Here's how the part is built. I have some questions about the finished solid (model axes, mm). Round coordinates to 2 decimals unless told otherwise and drop trailing zeros. Order: outer loops, then holes, each group sorted by start corner. A loop starts at its lowest first (then second) coordinate and runs counter-clockwise, first axis right, second up. Notation, with made-up numbers: (80.5, -17.5) - (93.5, -17.5) arc R21 ccw to (93.5, -9.5) - close; hole circle Ø6 at (82, 6.5). An arc over 180 degrees is marked (long way). Answer as a JSON object with one key per item and string values.
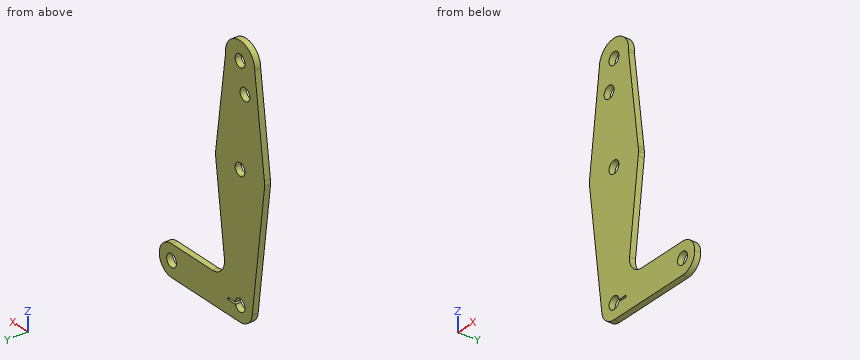
```python
from build123d import *

# Parameters (mm, degrees)
F0_R     = 3.175
F1_DEPTH = 3.048


with BuildPart() as f1:
    # F0 (on Front) → F1 (new body)
    with BuildSketch(Plane.XZ):
        with BuildLine():
            ThreePointArc((-9.525, 50.8), (-6.7351920908, 44.0648079092), (0, 41.275))
            ThreePointArc((0, 41.275), (6.3093081085, 43.6642970779), (9.4533014816, 49.6335026369))
            ThreePointArc((9.4533014816, 49.6335026369), (9.5070584728, 50.2156506234), (9.525, 50.8))
            ThreePointArc((9.525, 50.8), (0, 60.325), (-9.525, 50.8))
        make_face()
        with BuildLine():
            ThreePointArc((3.175, 50.8), (2.2450640303, 48.5549359697), (0, 47.625))
            ThreePointArc((0, 47.625), (-2.2450640303, 53.0450640303), (3.175, 50.8))
        make_face(mode=Mode.SUBTRACT)
        with BuildLine():
            ThreePointArc((9.4533014816, 49.6335026369), (6.3093081085, 43.6642970779), (0, 41.275))
            Line((0, 41.275), (0, 36.5252))
            Line((0, 36.5252), (0, 15.875))
            ThreePointArc((0, 15.875), (10.2323349377, 12.1373368876), (15.646399532, 2.6843633667))
            Line((15.646399532, 2.6843633667), (9.4533014816, 49.6335026369))
        make_face()
        with BuildLine():
            Line((0, 36.5252), (0, 41.275))
            ThreePointArc((0, 41.275), (-6.7351920908, 44.0648079092), (-9.525, 50.8))
            Line((-9.525, 50.8), (-15.7474569171, 2.008289233))
            ThreePointArc((-15.7474569171, 2.008289233), (-10.4912828917, 11.9142187443), (0, 15.875))
            Line((0, 15.875), (0, 36.5252))
        make_face()
        with Locations((-3.175, 36.5252)):
            Circle(F0_R, mode=Mode.SUBTRACT)
        with BuildLine():
            ThreePointArc((15.646399532, 2.6843633667), (10.2323349377, 12.1373368876), (0, 15.875))
            Line((0, 15.875), (0, 3.175))
            ThreePointArc((0, 3.175), (2.2450640303, 2.2450640303), (3.175, 0))
            ThreePointArc((3.175, 0), (2.2450640303, -2.2450640303), (0, -3.175))
            Line((0, -3.175), (0, -15.875))
            ThreePointArc((0, -15.875), (10.5003255684, -11.9062499536), (15.7504882912, -1.9843748607))
            ThreePointArc((15.7504882912, -1.9843748607), (15.8438414948, -0.9941386666), (15.875, 0))
            ThreePointArc((15.875, 0), (15.8580619796, 0.7331406754), (15.807284063, 1.4647168844))
            Line((15.807284063, 1.4647168844), (15.646399532, 2.6843633667))
        make_face()
        with BuildLine():
            Line((0, 3.175), (0, 15.875))
            ThreePointArc((0, 15.875), (-10.4912828917, 11.9142187443), (-15.7474569171, 2.008289233))
            ThreePointArc((-15.7474569171, 2.008289233), (-11.9142187443, -10.4912828917), (0, -15.875))
            Line((0, -15.875), (0, -3.175))
            ThreePointArc((0, -3.175), (-3.175, 0), (0, 3.175))
        make_face()
        with BuildLine():
            ThreePointArc((0, -15.875), (-11.9142187443, -10.4912828917), (-15.7474569171, 2.008289233))
            Line((-15.7474569171, 2.008289233), (-16.0035761028, 0))
            Line((-16.0035761028, 0), (-7.8751974831, -64.4925577322))
            ThreePointArc((-7.8751974831, -64.4925577322), (-5.9532484095, -58.2499771786), (0, -55.5625))
            Line((0, -55.5625), (0, -15.875))
        make_face()
        with BuildLine():
            ThreePointArc((15.807284063, 1.4647168844), (15.7386605945, 2.0760991524), (15.646399532, 2.6843633667))
            Line((15.646399532, 2.6843633667), (15.807284063, 1.4647168844))
        make_face()
        with BuildLine():
            ThreePointArc((15.7504882912, -1.9843748607), (10.5003255684, -11.9062499536), (0, -15.875))
            Line((0, -15.875), (0, -55.5625))
            ThreePointArc((0, -55.5625), (5.6126600757, -57.8873399243), (7.9375, -63.5))
            Line((7.9375, -63.5), (36.5125, -63.5))
            ThreePointArc((36.5125, -63.5), (38.8373399243, -57.8873399243), (44.45, -55.5625))
            Line((44.45, -55.5625), (18.0149584672, -55.5625))
            ThreePointArc((18.0149584672, -55.5625), (12.0523084668, -52.8708630179), (10.1271139399, -46.6185249989))
            Line((10.1271139399, -46.6185249989), (15.7504882912, -1.9843748607))
        make_face()
        with BuildLine():
            Line((16.0004960243, 0), (15.807284063, 1.4647168844))
            ThreePointArc((15.807284063, 1.4647168844), (15.8580619796, 0.7331406754), (15.875, 0))
            ThreePointArc((15.875, 0), (15.8438414948, -0.9941386666), (15.7504882912, -1.9843748607))
            Line((15.7504882912, -1.9843748607), (16.0004960243, 0))
        make_face()
        with BuildLine():
            Line((0, -60.325), (0, -55.5625))
            ThreePointArc((0, -55.5625), (-5.9532484095, -58.2499771786), (-7.8751974831, -64.4925577322))
            Line((-7.8751974831, -64.4925577322), (-3.0158670641, -64.4925577322))
            ThreePointArc((-3.0158670641, -64.4925577322), (-2.5721582183, -61.6386491196), (0, -60.325))
        make_face()
        with BuildLine():
            Line((-3.0158670641, -64.4925577322), (-7.8751974831, -64.4925577322))
            ThreePointArc((-7.8751974831, -64.4925577322), (-5.2500228214, -69.4532484095), (0, -71.4375))
            ThreePointArc((0, -71.4375), (5.2500228214, -69.4532484095), (7.8751974831, -64.4925577322))
            Line((7.8751974831, -64.4925577322), (3.0158670641, -64.4925577322))
            ThreePointArc((3.0158670641, -64.4925577322), (0, -66.675), (-3.0158670641, -64.4925577322))
        make_face()
        with BuildLine():
            Line((36.5125, -63.5), (7.9375, -63.5))
            ThreePointArc((7.9375, -63.5), (7.9219090588, -63.997255582), (7.8751974831, -64.4925577322))
            ThreePointArc((7.8751974831, -64.4925577322), (5.2500228214, -69.4532484095), (0, -71.4375))
            Line((0, -71.4375), (44.45, -71.4375))
            ThreePointArc((44.45, -71.4375), (38.8373399243, -69.1126600757), (36.5125, -63.5))
        make_face()
        with BuildLine():
            ThreePointArc((44.45, -55.5625), (38.8373399243, -57.8873399243), (36.5125, -63.5))
            ThreePointArc((36.5125, -63.5), (38.8373399243, -69.1126600757), (44.45, -71.4375))
            ThreePointArc((44.45, -71.4375), (50.0626600757, -69.1126600757), (52.3875, -63.5))
            ThreePointArc((52.3875, -63.5), (50.0626600757, -57.8873399243), (44.45, -55.5625))
        make_face()
        with BuildLine():
            ThreePointArc((47.625, -63.5), (44.45, -66.675), (41.275, -63.5))
            ThreePointArc((41.275, -63.5), (44.45, -60.325), (47.625, -63.5))
        make_face(mode=Mode.SUBTRACT)
        with BuildLine():
            ThreePointArc((7.9375, -63.5), (5.6126600757, -57.8873399243), (0, -55.5625))
            Line((0, -55.5625), (0, -60.325))
            ThreePointArc((0, -60.325), (2.2450640303, -61.2549359697), (3.175, -63.5))
            Line((3.175, -63.5), (7.9375, -63.5))
        make_face()
    extrude(amount=F1_DEPTH)


solid = f1.part
```
1. For P1, Ø1, axis at y = -2.5, z = -8, coming from the -X side; P2, Ø1, axis at x = 8.5, y = -1.5, coming from the +Z side; P3, Ø1.5, axis at y = -2.5, z = -44, coming from the +X side, each with a flat end and sliding along its axis, tell me the tip position at first contact or that it passes through.
Responses:
{"P1": "x = -15.06", "P2": "z = 55.97", "P3": "x = 10.55"}
2. If I drill on L1, parallel to X at y = -1.95, z = 50.8 (3 decimals); L2, parallel to Z at x = 44, y = -0.55; L3, parallel to Z at x = 4, y = -0.45, over which ranges is the centre line in solid material (lowest first)? Write a range as [from, to].
Responses:
{"L1": "[-9.525, -3.175], [3.175, 9.525]", "L2": "[-71.44, -66.64], [-60.36, -55.56]", "L3": "[-71.44, -64.49], [-63.5, 59.44]"}
3. Imagine slicing it at A-A (x = -5). List the corners of the cut face in (y, z) for me, plus the area to 3 significant figures.
Responses:
{"outline": "(-3.05, -69.66) - (0, -69.66) - (0, 33.93) - (-3.05, 33.93) - close; (-3.05, 39.12) - (0, 39.12) - (0, 58.91) - (-3.05, 58.91) - close", "area": "376 mm2"}
4. Imagine slicing it at B-B (y = -1.55). Give the number of separate pieces and of enclosed holes in the cut face, plus the area to 3 significant figures.
Responses:
{"separate pieces": "1", "enclosed holes": "5", "area": "3,600 mm2"}
5. Imagine slicing it at C-C (z = -43.5). List the corners of the cut face in (x, y) for me.
Responses:
{"outline": "(-10.52, -3.05) - (10.52, -3.05) - (10.52, 0) - (-10.52, 0) - close"}
6. Imagine slicing it at D-D (z = 19). List the corners of the cut face in (x, y) for me.
Responses:
{"outline": "(-13.58, -3.05) - (13.49, -3.05) - (13.49, 0) - (-13.58, 0) - close"}
